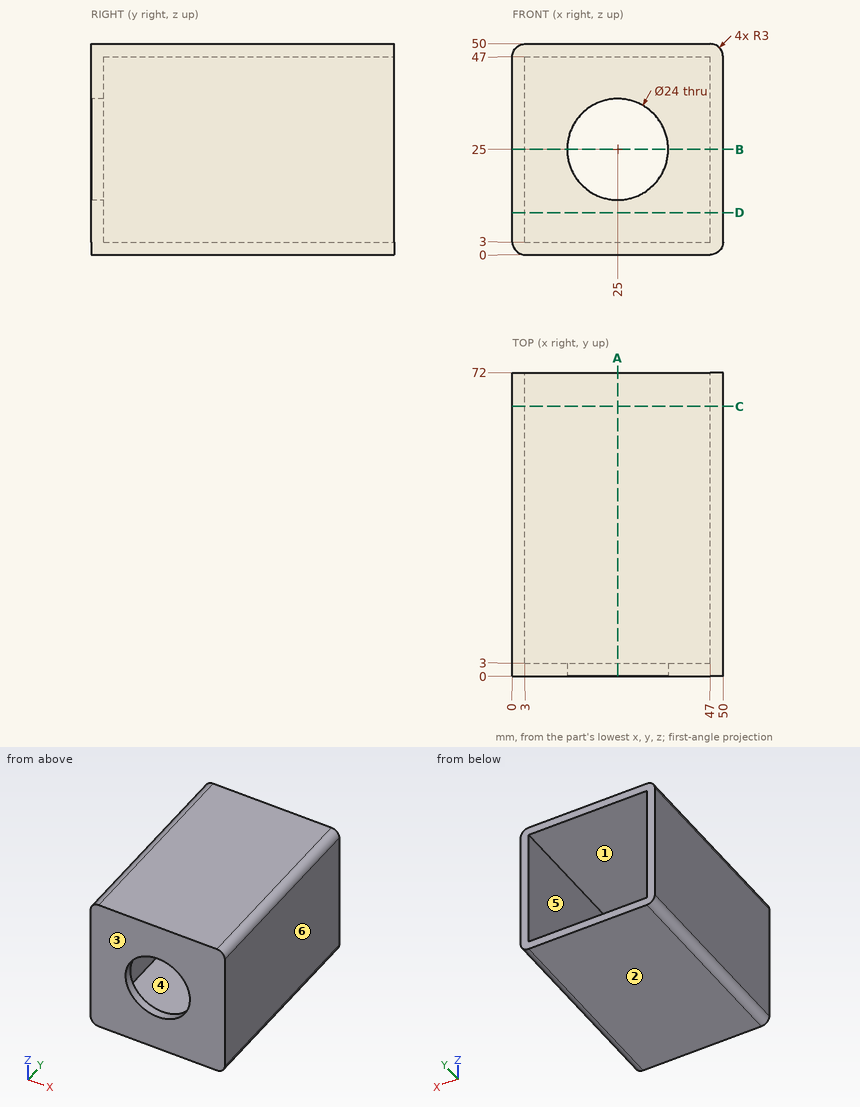
Print and shaded views of the part. All mm, measured from the part's lowest x, y and z. A direction names the side the tool comes from. Coordinates: 2 decimals unless noted, no trailing zeros. Write each loop counter-clockwise with the first axis right and the second up, starting at its lowest first coordinate (ties: lowest second). Pieces come first, ordered by that corner, then holes. Notation, with made-up numbers: M 75.5,23 L 107.5,23 A19 ccw 107.5,55 Z; hole C -12.5,-1.75 d11. An arc over 180 degrees is marked long. Return JSON: item names as keys, results as strings.
1. Probe L1, parallel to X at y = 41.5, z = 44; L2, parallel to X at y = 1.1, z = 25. List the from-to ranges inside material, lowest first.
Determined:
{"L1": "0 to 3, 47 to 50", "L2": "0 to 13, 37 to 50"}
2. 3-axis set-ups, long thin cutter, end or side, ignore diameter. For the marked faces 5 and 6: which of +Z, -Z, +X, -X, +Y, -Y reach the whole face in a straight line?
Determined:
{"face 5": "+Y", "face 6": "+Z, -Z, +X, +Y, -Y"}
3. Saw through at B-B, the plane z = 25. Write the cut outline in (x, y).
Determined:
{"outline": "M 0,0 L 13,0 L 13,3 L 3,3 L 3,72 L 0,72 Z; M 37,0 L 50,0 L 50,72 L 47,72 L 47,3 L 37,3 Z"}
4. Saw through at A-A, the plane x = 25. Write the cut outline in (y, z), then the cut area to 3 significant figures.
Determined:
{"outline": "M 0,0 L 72,0 L 72,3 L 3,3 L 3,13 L 0,13 Z; M 0,37 L 3,37 L 3,47 L 72,47 L 72,50 L 0,50 Z", "area": "492 mm²"}
5. Saw through at C-C, the plane y = 64. Write the cut outline in (x, z).
Determined:
{"outline": "M 0,3 A3 ccw 3,0 L 47,0 A3 ccw 50,3 L 50,47 A3 ccw 47,50 L 3,50 A3 ccw 0,47 Z; hole M 3,3 L 47,3 L 47,47 L 3,47 Z"}
6. Flat gauge pin, fed straight in: pin 1 Ø2 at (x, z) = (19.5, 12) entering from +Y. Where does the tip first touch, or does it go through?
Determined:
{"pin 1": "y = 3"}
7. Pull direction Z, two halves, no side cores. Call the marked faces 1, 2, 3 and 4: pulls with the +Z half, pulls with the -Z half, needs draft (parallel to the pull), parting line crosses it, or undercut.
Determined:
{"face 1": "undercut", "face 2": "pulls with the -Z half", "face 3": "needs draft", "face 4": "undercut"}
8. Saw through at D-D, the plane z = 10. Write the cut outline in (x, y), then the cut area to 3 significant figures.
Determined:
{"outline": "M 0,0 L 50,0 L 50,72 L 47,72 L 47,3 L 3,3 L 3,72 L 0,72 Z", "area": "564 mm²"}
